Check sheet for the modelled part. Datum: model origin and axes. Units: mm. Face numbers are marked on the shaded views. A direction names the side the tool comes from. Give positions to 0.01 mm unless a question says otherwise; leave off trailing zeros. Order: outer loops, then holes, each group sorted by start corner. A loop starts at its lowest first (then second) coordinate and runs counter-clockwise, first axis right, second up. Notation, with made-up numbers: M 54.5,26.25 L 90.5,26.25 A27 cw 90.5,59.25 Z; hole C 42.25,42.5 d1. An arc over 180 degrees is marked long. One line per question, with ' | ' between items. Start each with the question number.
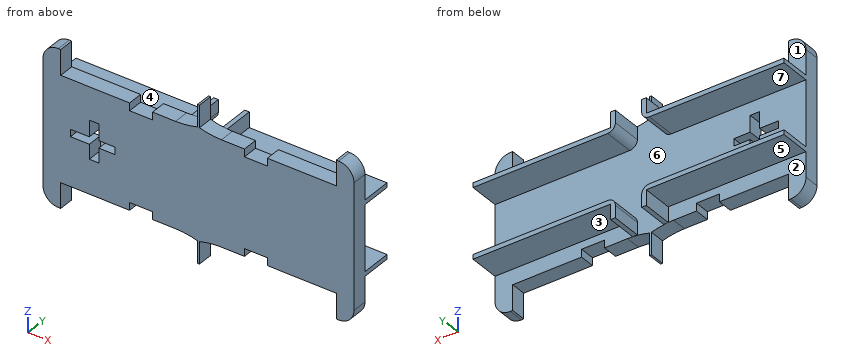
```python
from build123d import *

# Parameters (mm, degrees)
SKETCH1_W            = 203.2
SKETCH1_H            = 101.6
BOSS_EXTRUDE1_DEPTH  = 10
CUT_EXTRUDE1_DEPTH   = 115.031574575
MIRROR3_COPY_1_DEPTH = 115.031574575
FILLET2_R            = 10
FILLET3_R            = 10
FILLET4_R            = 10
FILLET5_R            = 10
CUT_EXTRUDE2_DEPTH   = 115.031574575
BOSS_EXTRUDE8_DEPTH  = 20
FILLET9_R            = 5
FILLET9_OF_MIRROR7_R = 5
MIRROR9_START        = 10
MIRROR9_DEPTH        = 20


# Read off the part's stored shape, not the designer's step: Mirror9
with BuildPart() as part:
    # Sketch1 → Boss-Extrude1 (new body)
    with BuildSketch(Plane(origin=(0, 0, 0), x_dir=(1, 0, 0), z_dir=(0, 1, 0))):
        Rectangle(SKETCH1_W, SKETCH1_H)
    extrude(amount=BOSS_EXTRUDE1_DEPTH)

    # Sketch4 → Cut-Extrude1 (cut, through all)
    with BuildSketch(Plane(origin=(0, 10, 0), x_dir=(1, 0, 0), z_dir=(0, 1, 0))):
        with BuildLine():
            Line((-30.016608914, 34.326781051), (-15.016608914, 34.326781051))
            ThreePointArc((-15.016608914, 34.326781051), (-7.755121488, 34.843235841), (-0.639820714, 36.382203056))
            Line((-0.639820714, 36.382203056), (-0.639820714, 56.908402461))
            Line((-0.639820714, 56.908402461), (-90.016608914, 56.908402461))
            Line((-90.016608914, 56.908402461), (-90.016608914, 34.326781051))
            Line((-90.016608914, 34.326781051), (-45.016608914, 34.326781051))
            Line((-45.016608914, 34.326781051), (-45.016608914, 29.326781051))
            Line((-45.016608914, 29.326781051), (-30.016608914, 29.326781051))
            Line((-30.016608914, 29.326781051), (-30.016608914, 34.326781051))
        make_face()
    cut_extrude1 = extrude(amount=-CUT_EXTRUDE1_DEPTH, mode=Mode.SUBTRACT)

    # Mirror2: Cut-Extrude1 across plane
    add(cut_extrude1.mirror(Plane.XY), mode=Mode.SUBTRACT)

    # Mirror3: Cut-Extrude1 across plane
    add(cut_extrude1.mirror(Plane(origin=(0, 0, 0), x_dir=(0, 0, 1), z_dir=(1, 0, 0))), mode=Mode.SUBTRACT)

    # Mirror3 copy 1 sketch → Mirror3 copy 1 (cut, through all)
    with BuildSketch(Plane(origin=(0, 10, 0), x_dir=(-1, 0, 0), z_dir=(0, 1, 0))):
        with BuildLine():
            Line((-30.016608914, 34.326781051), (-15.016608914, 34.326781051))
            ThreePointArc((-15.016608914, 34.326781051), (-7.755121488, 34.843235841), (-0.639820714, 36.382203056))
            Line((-0.639820714, 36.382203056), (-0.639820714, 56.908402461))
            Line((-0.639820714, 56.908402461), (-90.016608914, 56.908402461))
            Line((-90.016608914, 56.908402461), (-90.016608914, 34.326781051))
            Line((-90.016608914, 34.326781051), (-45.016608914, 34.326781051))
            Line((-45.016608914, 34.326781051), (-45.016608914, 29.326781051))
            Line((-45.016608914, 29.326781051), (-30.016608914, 29.326781051))
            Line((-30.016608914, 29.326781051), (-30.016608914, 34.326781051))
        make_face()
    extrude(amount=-MIRROR3_COPY_1_DEPTH, mode=Mode.SUBTRACT)

    # Fillet2
    fillet2_edges = [part.edges().sort_by_distance(p)[0] for p in [
        (-101.6, 5, 50.8),
    ]]
    fillet(fillet2_edges, radius=FILLET2_R)

    # Fillet3
    fillet3_edges = [part.edges().sort_by_distance(p)[0] for p in [
        (-101.6, 5, -50.8),
    ]]
    fillet(fillet3_edges, radius=FILLET3_R)

    # Fillet4
    fillet4_edges = [part.edges().sort_by_distance(p)[0] for p in [
        (101.6, 5, -50.8),
    ]]
    fillet(fillet4_edges, radius=FILLET4_R)

    # Fillet5
    fillet5_edges = [part.edges().sort_by_distance(p)[0] for p in [
        (101.6, 5, 50.8),
    ]]
    fillet(fillet5_edges, radius=FILLET5_R)

    # Sketch6 → Cut-Extrude2 (cut, through all)
    with BuildSketch(Plane(origin=(0, 10, 0), x_dir=(1, 0, 0), z_dir=(0, 1, 0))):
        Polygon((-65.154466358, 2.427920334), (-54.461184026, 2.427920334), (-54.461184026, -2.324649591), (-65.154466358, -2.324649591), (-65.154466358, -13.017931923), (-71.33280726, -13.017931923), (-71.33280726, -2.324649591), (-83.689489065, -2.324649591), (-83.689489065, 2.427920334), (-71.33280726, 2.427920334), (-71.33280726, 11.982068077), (-65.154466358, 11.982068077), align=None)
    extrude(amount=-CUT_EXTRUDE2_DEPTH, mode=Mode.SUBTRACT)

    # Sketch11 → Boss-Extrude8 (add)
    with BuildSketch(Plane(origin=(0, 10, 0), x_dir=(1, 0, 0), z_dir=(0, 1, 0))):
        Polygon((-101.6, 24.424351811), (-11.6, 24.424351811), (-11.6, 34.440665029), (-8.6, 34.440665029), (-8.6, 21.424351811), (-101.6, 21.424351811), align=None)
    boss_extrude8 = extrude(amount=BOSS_EXTRUDE8_DEPTH)

    # Fillet9
    fillet9_edges = [part.edges().sort_by_distance(p)[0] for p in [
        (-8.6, 20, -21.424351811),
    ]]
    fillet(fillet9_edges, radius=FILLET9_R)

    # Mirror7: Boss-Extrude8 across plane
    add(boss_extrude8.mirror(Plane.XY))

    # Fillet9 of Mirror7
    fillet9_of_mirror7_edges = [part.edges().sort_by_distance(p)[0] for p in [
        (-8.6, 20, 21.424351811),
    ]]
    fillet(fillet9_of_mirror7_edges, radius=FILLET9_OF_MIRROR7_R)

    # Mirror9 outline → Mirror9 (add)
    with BuildSketch(Plane(origin=(0, 0, 0), x_dir=(1, 0, 0), z_dir=(0, 1, 0)).offset(MIRROR9_START)):
        with BuildLine():
            Line((11.6, 24.424351811), (11.6, 34.440665029))
            Line((11.6, 34.440665029), (8.6, 34.440665029))
            Line((8.6, 34.440665029), (8.6, 26.424351811))
            ThreePointArc((8.6, 26.424351811), (10.064466094, 22.888817905), (13.6, 21.424351811))
            Line((13.6, 21.424351811), (101.6, 21.424351811))
            Line((101.6, 21.424351811), (101.6, 24.424351811))
            Line((101.6, 24.424351811), (11.6, 24.424351811))
        make_face()
        with BuildLine():
            Line((101.6, -24.424351811), (101.6, -21.424351811))
            Line((101.6, -21.424351811), (13.6, -21.424351811))
            ThreePointArc((13.6, -21.424351811), (10.064466094, -22.888817905), (8.6, -26.424351811))
            Line((8.6, -26.424351811), (8.6, -34.440665029))
            Line((8.6, -34.440665029), (11.6, -34.440665029))
            Line((11.6, -34.440665029), (11.6, -24.424351811))
            Line((11.6, -24.424351811), (101.6, -24.424351811))
        make_face()
    extrude(amount=MIRROR9_DEPTH)


solid = part.part
```
Item 1: Scan lines: probe 1 along X at (y, z) = (4, 36.5); probe 2 along X at (y, z) = (4.75, -7); probe 3 along Z at (x, y) = (88, 24.5). Record each from-to range of solid material in increasing order. Write a range as [from, to].
Item 2: Section check C-C, the plane x = 41. Record the cut outline in (y, z).
Item 3: Section check B-B, the plane z = 44. Record the cut outline in (x, y), then the cut area to 3 significant figures.
Item 4: Section check D-D, the plane x = -23.5. Record the cut outline in (y, z), then the cut area to 3 significant figures.
Item 5: Draft check along Z on the marked faces 4, 5, 6 and 7. Enter one of: released by +Z, released by -Z, zero draft, split by the parting line, or undercut.
Item 6: Go/stop test with flat-tipped pins: P1, Ø2, axis at x = 58.5, z = 7.5, coming from the -Y side; P2, Ø5, axis at x = 40.5, y = 3.5, coming from the +Z side; P3, Ø1, axis at x = -39, y = 25, coming from the -Z side; P4, Ø10, axis at y = 16, z = -8.5, coming from the -X side. Record where each tip stops, or that it passes through.
Item 7: Section check A-A, the plane y = 17.5. Record the cut outline in (x, z), then the cut area to 3 significant figures.
Item 8: Set-up check for the marked faces 1, 2 and 3: record each of +Z, -Z, +X, -X, +Y, -Y from which the full face is reachable in a straight line by a thin tool's end or side.
Reported:
1) probe 1: x = [-101.6, -90.02], [-0.64, 0.64], [90.02, 101.6] | probe 2: x = [-101.6, -71.33], [-65.15, 101.6] | probe 3: z = [-24.42, -21.42], [21.42, 24.42]
2) outline: M 0,-29.33 L 10,-29.33 L 10,-24.42 L 30,-24.42 L 30,-21.42 L 10,-21.42 L 10,21.42 L 30,21.42 L 30,24.42 L 10,24.42 L 10,29.33 L 0,29.33 Z
3) outline: M -101.07,0 L -90.02,0 L -90.02,10 L -101.07,10 Z; M -0.64,0 L 0.64,0 L 0.64,10 L -0.64,10 Z; M 90.02,0 L 101.07,0 L 101.07,10 L 90.02,10 Z | area: 234 mm^2
4) outline: M 0,-34.33 L 10,-34.33 L 10,-24.42 L 30,-24.42 L 30,-21.42 L 10,-21.42 L 10,21.42 L 30,21.42 L 30,24.42 L 10,24.42 L 10,34.33 L 0,34.33 Z | area: 807 mm^2
5) face 4: released by +Z | face 5: released by -Z | face 6: undercut | face 7: undercut
6) P1: stops at y = 0 | P2: stops at z = 29.33 | P3: stops at z = -24.42 | P4: passes through
7) outline: M -101.6,-24.42 L -11.6,-24.42 L -11.6,-34.44 L -8.6,-34.44 L -8.6,-26.42 A5 ccw -13.6,-21.42 L -101.6,-21.42 Z; M -101.6,21.42 L -13.6,21.42 A5 ccw -8.6,26.42 L -8.6,34.44 L -11.6,34.44 L -11.6,24.42 L -101.6,24.42 Z; M 8.6,-34.44 L 11.6,-34.44 L 11.6,-24.42 L 101.6,-24.42 L 101.6,-21.42 L 13.6,-21.42 A5 ccw 8.6,-26.42 Z; M 8.6,26.42 A5 ccw 13.6,21.42 L 101.6,21.42 L 101.6,24.42 L 11.6,24.42 L 11.6,34.44 L 8.6,34.44 Z | area: 1,210 mm^2
8) face 1: +Z, -X, +Y | face 2: -Z, -X, +Y | face 3: -Z, +X, +Y
